```python
from build123d import *

# Parameters (mm, degrees)
F1_DEPTH   = 5
F2_R       = 2
F3_DEPTH   = 25
F4_SIZE2   = 0.4330127019
F4_SIZE    = 0.75
F4_2_SIZE2 = 0.4330127019
F4_2_SIZE  = 0.75
F4_3_SIZE2 = 0.4330127019
F4_3_SIZE  = 0.75
F4_4_SIZE2 = 0.4330127019
F4_4_SIZE  = 0.75
F4_5_SIZE2 = 0.4330127019
F4_5_SIZE  = 0.75
F6_DEPTH   = 2.5


with BuildPart() as f1:
    # F0 (on Top) → F1 (new body)
    with BuildSketch(Plane.XY):
        with BuildLine():
            Line((79.5, -10), (79.5, 0))
            ThreePointArc((79.5, 0), (76.6326218032, 21.1587163024), (68.2373264008, 40.7911422452))
            ThreePointArc((68.2373264008, 40.7911422452), (65.5381568249, 45), (62.5797484655, 49.0308584668))
            ThreePointArc((62.5797484655, 49.0308584668), (37.0331769321, 70.3476638298), (5, 79.3426115023))
            ThreePointArc((5, 79.3426115023), (0, 79.5), (-5, 79.3426115023))
            ThreePointArc((-5, 79.3426115023), (-37.0331769321, 70.3476638298), (-62.5797484655, 49.0308584668))
            ThreePointArc((-62.5797484655, 49.0308584668), (-65.5381568249, 45), (-68.2373264008, 40.7911422452))
            ThreePointArc((-68.2373264008, 40.7911422452), (-76.6326218032, 21.1587163024), (-79.5, 0))
            Line((-79.5, 0), (-79.5, -10))
            Line((-79.5, -10), (-70.5, -10))
            Line((-70.5, -10), (-70.5, 0))
            ThreePointArc((-70.5, 0), (0, 70.5), (70.5, 0))
            Line((70.5, 0), (70.5, -10))
            Line((70.5, -10), (79.5, -10))
        make_face()
        with BuildLine():
            ThreePointArc((79.5, -10), (84.5, -5), (79.5, 0))
            Line((79.5, 0), (79.5, -10))
        make_face()
        with BuildLine():
            ThreePointArc((62.5797484655, 49.0308584668), (65.5381568249, 45), (68.2373264008, 40.7911422452))
            ThreePointArc((68.2373264008, 40.7911422452), (69.6600534805, 47.8301886792), (62.5797484655, 49.0308584668))
        make_face()
        with BuildLine():
            ThreePointArc((-5, 79.3426115023), (0, 79.5), (5, 79.3426115023))
            ThreePointArc((5, 79.3426115023), (0, 84.3426115023), (-5, 79.3426115023))
        make_face()
        with BuildLine():
            ThreePointArc((-68.2373264008, 40.7911422452), (-65.5381568249, 45), (-62.5797484655, 49.0308584668))
            ThreePointArc((-62.5797484655, 49.0308584668), (-69.6600534805, 47.8301886792), (-68.2373264008, 40.7911422452))
        make_face()
        with BuildLine():
            ThreePointArc((-79.5, 0), (-84.5, -5), (-79.5, -10))
            Line((-79.5, -10), (-79.5, 0))
        make_face()
    extrude(amount=F1_DEPTH)

    # F2 (on face) → F3 (cut)
    with BuildSketch(Plane.XY.offset(5)):
        with Locations((0, 79.3426115023)):
            Circle(F2_R)
        with Locations((-65.5381568249, 45)):
            Circle(F2_R)
        with Locations((65.5381568249, 45)):
            Circle(F2_R)
        with Locations((-79.5, -5)):
            Circle(F2_R)
        with Locations((79.5, -5)):
            Circle(F2_R)
    extrude(amount=-F3_DEPTH, mode=Mode.SUBTRACT)

    # F4
    f4_edges = [f1.edges().sort_by_distance(p)[0] for p in [
        (0, 70.5, 5),
    ]]
    f4_side = f1.faces().sort_by_distance((0, 70.5, 2.5))[0]
    chamfer(f4_edges, length=F4_SIZE, length2=F4_SIZE2, reference=f4_side)

    # F4#2
    f4_2_edges = [f1.edges().sort_by_distance(p)[0] for p in [
        (-37.033177, 70.347664, 5),
    ]]
    f4_2_side = f1.faces().sort_by_distance((-37.033177, 70.347664, 2.5))[0]
    chamfer(f4_2_edges, length=F4_2_SIZE, length2=F4_2_SIZE2, reference=f4_2_side)

    # F4#3
    f4_3_edges = [f1.edges().sort_by_distance(p)[0] for p in [
        (37.033177, 70.347664, 5),
    ]]
    f4_3_side = f1.faces().sort_by_distance((37.033177, 70.347664, 2.5))[0]
    chamfer(f4_3_edges, length=F4_3_SIZE, length2=F4_3_SIZE2, reference=f4_3_side)

    # F4#4
    f4_4_edges = [f1.edges().sort_by_distance(p)[0] for p in [
        (76.632622, 21.158716, 5),
    ]]
    f4_4_side = f1.faces().sort_by_distance((76.632622, 21.158716, 2.5))[0]
    chamfer(f4_4_edges, length=F4_4_SIZE, length2=F4_4_SIZE2, reference=f4_4_side)

    # F4#5
    f4_5_edges = [f1.edges().sort_by_distance(p)[0] for p in [
        (-76.632622, 21.158716, 5),
    ]]
    f4_5_side = f1.faces().sort_by_distance((-76.632622, 21.158716, 2.5))[0]
    chamfer(f4_5_edges, length=F4_5_SIZE, length2=F4_5_SIZE2, reference=f4_5_side)

    # F5 (on face) → F6 (cut)
    with BuildSketch(Plane(origin=(0, 0, 0), x_dir=(1, 0, 0), z_dir=(0, 0, -1))):
        with BuildLine():
            ThreePointArc((-79.5, 10), (-84.5, 5), (-79.5, 0))
            Line((-79.5, 0), (-70.5, 0))
            Line((-70.5, 0), (-70.5, 10))
            Line((-70.5, 10), (-79.5, 10))
        make_face()
        with BuildLine():
            Line((70.5, 0), (79.5, 0))
            ThreePointArc((79.5, 0), (84.5, 5), (79.5, 10))
            Line((79.5, 10), (70.5, 10))
            Line((70.5, 10), (70.5, 0))
        make_face()
    extrude(amount=-F6_DEPTH, mode=Mode.SUBTRACT)


solid = f1.part
```
Model file for the job. Use its own axes, mm. A direction names the side the tool comes from. Give positions to 0.01 mm unless a question says otherwise; leave off trailing zeros. Order: outer loops, then holes, each group sorted by start corner. A loop starts at its lowest first (then second) coordinate and runs counter-clockwise, first axis right, second up.
1) Saw through at B-B, the plane y = -5. Write the cut outline in (x, z).
2) Saw through at A-A, the plane x = 0. Write the cut outline in (y, z).
3) Wall check: probe 1 along X at (y, z) = (1.5, 2.8); probe 2 along X at (y, z) = (-5.5, 3.4); probe 3 along X at (y, z) = (58, 1.95). Give the ranges that are in metal, low to high.
4) Saw through at C-C, the plane y = 45. Count the separate pieces of the cut face and the enclosed holes in it, then the cut area to 3 significant figures.
5) Mould opens along Y. For faces 1 (the conical face through (-36.474, 70.284, 4.797)), 2 (the flat face through (0, 72, 5)), 3 (the cylindrical face through (-77.592, -4.399, 3.768)) say: +Y half, -Y half, draft (parallel to the pull), parting line (faces both ways), or undercut.
6) Pin check, flat tips, straight feed: pin 1 (2 mm diameter, centred on x = -55.5, y = 41.5, fed in from +Z); pin 2 (2 mm diameter, centred on x = 77, z = 0.5, fed in from -Y); pin 3 (1 mm diameter, centred on y = 5.5, z = 2.5, fed in from +X); pin 4 (2 mm diameter, centred on y = 30, z = 2, fed in from +X). Stop position of each tip, or through.
7) 3-axis set-ups, long thin cutter, end or side, ignore diameter. For faces 4 (the flat face through (77, -5, 2.5)), 5 (the cylindrical face through (-1.55, 70.483, 2.095)): which of +Z, -Z, +X, -X, +Y, -Y reach the whole face in a straight line?
Computed:
1. outline: (-84.5, 2.5) - (-81.5, 2.5) - (-81.5, 5) - (-84.5, 5) - close; (-77.5, 2.5) - (-70.5, 2.5) - (-70.5, 4.25) - (-70.93, 5) - (-77.5, 5) - close; (70.5, 2.5) - (77.5, 2.5) - (77.5, 5) - (70.93, 5) - (70.5, 4.25) - close; (81.5, 2.5) - (84.5, 2.5) - (84.5, 5) - (81.5, 5) - close
2. outline: (70.5, 0) - (77.34, 0) - (77.34, 5) - (70.93, 5) - (70.5, 4.25) - close; (81.34, 0) - (84.34, 0) - (84.34, 5) - (81.34, 5) - close
3. probe 1: x = -79.49 to -70.48, 70.48 to 79.49
3. probe 2: x = -84.47 to -81.44, -77.56 to -70.5, 70.5 to 77.56, 81.44 to 84.47
3. probe 3: x = -54.37 to -40.08, 40.08 to 54.37
4. separate pieces: 4
4. enclosed holes: 0
4. area: 122 mm2
5. face 1: +Y half
5. face 2: draft
5. face 3: undercut
6. pin 1: passes through
6. pin 2: stops at y = 0
6. pin 3: stops at x = 79.34
6. pin 4: stops at x = 74.02
7. face 4: -Z, +X, -X, -Y
7. face 5: +Z, -Z, -Y
